```python
from build123d import *

# Parameters (mm, degrees)
SKETCH1_W                      = 60
SKETCH1_H                      = 375.5
BASE_FLANGE1_DEPTH             = 4
EDGE_FLANGE1_STRIP_W           = 18
EDGE_FLANGE1_STRIP_H           = 4
EDGE_FLANGE1_STRIP_CUT_DEPTH   = 375.5
EDGE_FLANGE1_DEPTH             = 375.5
EDGE_FLANGE2_STRIP_W           = 18
EDGE_FLANGE2_STRIP_H           = 4
EDGE_FLANGE2_STRIP_CUT_DEPTH   = 55
EDGE_FLANGE2_STRIP_2_W         = 18
EDGE_FLANGE2_STRIP_2_H         = 4
EDGE_FLANGE2_STRIP_CUT_2_DEPTH = 55
EDGE_FLANGE2_STRIP_3_W         = 18
EDGE_FLANGE2_STRIP_3_H         = 4
EDGE_FLANGE2_STRIP_CUT_3_DEPTH = 55
EDGE_FLANGE2_STRIP_4_W         = 18
EDGE_FLANGE2_STRIP_4_H         = 4
EDGE_FLANGE2_STRIP_CUT_4_DEPTH = 55
EDGE_FLANGE2_DEPTH             = 55
EDGE_FLANGE2_BEND_DEPTH        = 55
EDGE_FLANGE2_BEND_2_DEPTH      = 55
EDGE_FLANGE2_BEND_3_DEPTH      = 55
SKETCH18_R                     = 4.6
EXTRUDE1_DEPTH                 = 386.948506928
SKETCH19_R                     = 4.6
EXTRUDE2_DEPTH                 = 4
SKETCH20_R                     = 4.6
EXTRUDE3_DEPTH                 = 4


# Sheet-metal steps are written as plain solids
with BuildPart() as part:
    # Sketch1 → Base-Flange1 (new body)
    with BuildSketch(Plane(origin=(0, 0, 0), x_dir=(1, 0, 0), z_dir=(0, 1, 0))):
        Rectangle(SKETCH1_W, SKETCH1_H)
    extrude(amount=BASE_FLANGE1_DEPTH)

    # Edge-Flange1 strip (across the edge) → Edge-Flange1 strip cut (cut)
    with BuildSketch(Plane(origin=(-30, 4, -187.75), x_dir=(1, 0, 0), z_dir=(0, 0, 1))):
        with Locations((-4, -2)):
            Rectangle(EDGE_FLANGE1_STRIP_W, EDGE_FLANGE1_STRIP_H)
    extrude(amount=EDGE_FLANGE1_STRIP_CUT_DEPTH, mode=Mode.SUBTRACT)

    # Edge-Flange1 section (across the edge) → Edge-Flange1 (add)
    with BuildSketch(Plane(origin=(-30, 4, -187.75), x_dir=(1, 0, 0), z_dir=(0, 0, 1))):
        with BuildLine():
            Line((0, 1), (0, 56))
            Line((0, 56), (4, 56))
            Line((4, 56), (4, 1))
            ThreePointArc((4, 1), (4.292893219, 0.292893219), (5, 0))
            Line((5, 0), (5, -4))
            ThreePointArc((5, -4), (1.464466094, -2.535533906), (0, 1))
        make_face()
    extrude(amount=EDGE_FLANGE1_DEPTH)

    # Edge-Flange2 strip (across the edge) → Edge-Flange2 strip cut (cut)
    with BuildSketch(Plane(origin=(-30, 5, 187.75), x_dir=(0, 0, -1), z_dir=(0, 1, 0))):
        with Locations((-4, -2)):
            Rectangle(EDGE_FLANGE2_STRIP_W, EDGE_FLANGE2_STRIP_H)
    extrude(amount=EDGE_FLANGE2_STRIP_CUT_DEPTH, mode=Mode.SUBTRACT)

    # Edge-Flange2 strip 2 (across the edge) → Edge-Flange2 strip cut 2 (cut)
    with BuildSketch(Plane(origin=(30, 0, 187.75), x_dir=(0, 0, -1), z_dir=(-1, 0, 0))):
        with Locations((-4, -2)):
            Rectangle(EDGE_FLANGE2_STRIP_2_W, EDGE_FLANGE2_STRIP_2_H)
    extrude(amount=EDGE_FLANGE2_STRIP_CUT_2_DEPTH, mode=Mode.SUBTRACT)

    # Edge-Flange2 strip 3 (across the edge) → Edge-Flange2 strip cut 3 (cut)
    with BuildSketch(Plane(origin=(-30, 60, -187.75), x_dir=(0, 0, 1), z_dir=(0, -1, 0))):
        with Locations((-4, -2)):
            Rectangle(EDGE_FLANGE2_STRIP_3_W, EDGE_FLANGE2_STRIP_3_H)
    extrude(amount=EDGE_FLANGE2_STRIP_CUT_3_DEPTH, mode=Mode.SUBTRACT)

    # Edge-Flange2 strip 4 (across the edge) → Edge-Flange2 strip cut 4 (cut)
    with BuildSketch(Plane(origin=(-25, 0, -187.75), x_dir=(0, 0, 1), z_dir=(1, 0, 0))):
        with Locations((-4, -2)):
            Rectangle(EDGE_FLANGE2_STRIP_4_W, EDGE_FLANGE2_STRIP_4_H)
    extrude(amount=EDGE_FLANGE2_STRIP_CUT_4_DEPTH, mode=Mode.SUBTRACT)

    # Edge-Flange2 section (across the edge) → Edge-Flange2 (add)
    with BuildSketch(Plane(origin=(-30, 5, 187.75), x_dir=(0, 0, -1), z_dir=(0, 1, 0))):
        with BuildLine():
            Line((0, 1), (0, 36))
            Line((0, 36), (4, 36))
            Line((4, 36), (4, 1))
            ThreePointArc((4, 1), (4.292893219, 0.292893219), (5, 0))
            Line((5, 0), (5, -4))
            ThreePointArc((5, -4), (1.464466094, -2.535533906), (0, 1))
        make_face()
    extrude(amount=EDGE_FLANGE2_DEPTH)

    # Edge-Flange2 section 2 (across the edge) → Edge-Flange2 bend (add)
    with BuildSketch(Plane(origin=(30, 0, 187.75), x_dir=(0, 0, -1), z_dir=(-1, 0, 0))):
        with BuildLine():
            Line((0, 1), (0, 36))
            Line((0, 36), (4, 36))
            Line((4, 36), (4, 1))
            ThreePointArc((4, 1), (4.292893219, 0.292893219), (5, 0))
            Line((5, 0), (5, -4))
            ThreePointArc((5, -4), (1.464466094, -2.535533906), (0, 1))
        make_face()
    extrude(amount=EDGE_FLANGE2_BEND_DEPTH)

    # Edge-Flange2 section 3 (across the edge) → Edge-Flange2 bend 2 (add)
    with BuildSketch(Plane(origin=(-30, 60, -187.75), x_dir=(0, 0, 1), z_dir=(0, -1, 0))):
        with BuildLine():
            Line((0, 1), (0, 36))
            Line((0, 36), (4, 36))
            Line((4, 36), (4, 1))
            ThreePointArc((4, 1), (4.292893219, 0.292893219), (5, 0))
            Line((5, 0), (5, -4))
            ThreePointArc((5, -4), (1.464466094, -2.535533906), (0, 1))
        make_face()
    extrude(amount=EDGE_FLANGE2_BEND_2_DEPTH)

    # Edge-Flange2 section 4 (across the edge) → Edge-Flange2 bend 3 (add)
    with BuildSketch(Plane(origin=(-25, 0, -187.75), x_dir=(0, 0, 1), z_dir=(1, 0, 0))):
        with BuildLine():
            Line((0, 1), (0, 36))
            Line((0, 36), (4, 36))
            Line((4, 36), (4, 1))
            ThreePointArc((4, 1), (4.292893219, 0.292893219), (5, 0))
            Line((5, 0), (5, -4))
            ThreePointArc((5, -4), (1.464466094, -2.535533906), (0, 1))
        make_face()
    extrude(amount=EDGE_FLANGE2_BEND_3_DEPTH)

    # Sketch18 → Extrude1 (cut, through all)
    with BuildSketch(Plane.XY.offset(187.75)):
        with Locations((-46, 47.5)):
            Circle(SKETCH18_R)
        with Locations((-46, 17.5)):
            Circle(SKETCH18_R)
        with Locations((-12.5, -16)):
            Circle(SKETCH18_R)
        with Locations((17.5, -16)):
            Circle(SKETCH18_R)
    extrude(amount=-EXTRUDE1_DEPTH, mode=Mode.SUBTRACT)

    # Sketch19 → Extrude2 (cut)
    with BuildSketch(Plane(origin=(-26, 0, 0), x_dir=(0, 0, -1), z_dir=(1, 0, 0))):
        with Locations(Location((-107.75, 35, 0), (0, 0, 90))):
            Circle(SKETCH19_R)
        with Locations(Location((107.75, 35, 0), (0, 0, 90))):
            Circle(SKETCH19_R)
    extrude(amount=-EXTRUDE2_DEPTH, mode=Mode.SUBTRACT)

    # Sketch20 → Extrude3 (cut)
    with BuildSketch(Plane(origin=(0, 4, 0), x_dir=(1, 0, 0), z_dir=(0, 1, 0))):
        with Locations(Location((5, 107.75, 0), (0, 0, 270))):
            Circle(SKETCH20_R)
        with Locations(Location((5, -107.75, 0), (0, 0, 270))):
            Circle(SKETCH20_R)
    extrude(amount=-EXTRUDE3_DEPTH, mode=Mode.SUBTRACT)


solid = part.part
```
Model file for the job. Use its own axes, mm. A direction names the side the tool comes from. Coordinates: 2 decimals unless noted, no trailing zeros. Loops run counter-clockwise (first coordinate to the right, second up) from the corner with the lowest first, then second, coordinate; pieces in that order, holes last. Notation, with made-up numbers: (2, 74.5) - (23, 74.5) arc R13 cw to (23, 87.5) - close; hole circle Ø7 at (-12, -6.75). An arc over 180 degrees is marked (long way). Answer as a JSON object with one key per item and string values. Group by question number.
(1) Two-plate mould, pull along Y, no slides. Class faces 1 (the face through (-27.972, 37.123, -111.831)), 2 (the face through (-49, 33, -183.75)), 3 (the face through (-28, 60, 1)), 4 (the face through (-43.53, 21.38, -185.72)): released by +Y, released by -Y, zero draft, split by the parting line, or undercut.
(2) Flat gauge pins, fed straight in: pin 1 (12 mm diameter, centred on y = 35, z = 107.75, fed in from +X); pin 2 (1.5 mm diameter, centred on y = -11.5, z = -185.5, fed in from -X); pin 3 (3 mm diameter, centred on x = -18.5, z = 128.5, fed in from -Y). Where does each tip first touch, or does it go through?
(3) Cut at D-D (y = 17.5). Give the cut face in (x, z), then the cut area to 3 significant figures.
(4) Cut at C-C (x = -12.5). Give the cut face in (y, z), then the cut area to 3 significant figures.
(5) Tool access for faces 5 (the face through (-49, 32, 183.75)), 6 (the face through (-10.03, -12.12, 185.78)), 7 (the face through (2, 0, -3)): list every direction of +Z, -Z, +X, -X, +Y, -Y with a clear straight run to the whole face (end or side of a thin tool).
(6) Probe line 1 along Y through (x, z) = (-46, -185.95); line 2 along Z through (x, y) = (-9, -21); line 3 along X through (y, z) = (9, 117). List the from-to ranges inside material, lowest first.
(7) Cut at B-B (z = -107.75). Give the cut face in (x, y).
(8) Cut at A-A (y = -16). Give the cut face in (x, z), then the cut area to 3 significant figures.
Geometry says:
{
 "1": {"face 1": "undercut", "face 2": "zero draft", "face 3": "released by +Y", "face 4": "undercut"},
 "2": {"pin 1": "stops at x = -26", "pin 2": "stops at x = -25", "pin 3": "stops at y = 0"},
 "3": {"outline": "(-66, -187.75) - (-50.6, -187.75) - (-50.6, -183.75) - (-66, -183.75) - close; (-66, 183.75) - (-50.6, 183.75) - (-50.6, 187.75) - (-66, 187.75) - close; (-41.4, -187.75) - (-31, -187.75) arc R5 ccw to (-26, -182.75) - (-26, 182.75) arc R5 ccw to (-31, 187.75) - (-41.4, 187.75) - (-41.4, 183.75) - (-31, 183.75) arc R1 cw to (-30, 182.75) - (-30, -182.75) arc R1 cw to (-31, -183.75) - (-41.4, -183.75) - close", "area": "1,710 mm^2"},
 "4": {"outline": "(-36, -187.75) - (-20.6, -187.75) - (-20.6, -183.75) - (-36, -183.75) - close; (-36, 183.75) - (-20.6, 183.75) - (-20.6, 187.75) - (-36, 187.75) - close; (-11.4, -187.75) - (-1, -187.75) arc R5 ccw to (4, -182.75) - (4, 182.75) arc R5 ccw to (-1, 187.75) - (-11.4, 187.75) - (-11.4, 183.75) - (-1, 183.75) arc R1 cw to (0, 182.75) - (0, -182.75) arc R1 cw to (-1, -183.75) - (-11.4, -183.75) - close", "area": "1,710 mm^2"},
 "5": {"face 5": "-X, +Y, -Y", "face 6": "+Z, -Z", "face 7": "+X, -X, -Y"},
 "6": {"line 1": "y = 5 to 12.9, 22.1 to 42.9, 52.1 to 60", "line 2": "z = -187.75 to -183.75, 183.75 to 187.75", "line 3": "x = -30 to -26"},
 "7": {"outline": "(-30, 5) arc R5 ccw to (-25, 0) - (0.4, 0) - (0.4, 4) - (-25, 4) arc R1 cw to (-26, 5) - (-26, 30.4) - (-30, 30.4) - close; (-30, 39.6) - (-26, 39.6) - (-26, 60) - (-30, 60) - close; (9.6, 0) - (30, 0) - (30, 4) - (9.6, 4) - close"},
 "8": {"outline": "(-25, -187.75) - (-17.1, -187.75) - (-17.1, -183.75) - (-25, -183.75) - close; (-25, 183.75) - (-17.1, 183.75) - (-17.1, 187.75) - (-25, 187.75) - close; (-7.9, -187.75) - (12.9, -187.75) - (12.9, -183.75) - (-7.9, -183.75) - close; (-7.9, 183.75) - (12.9, 183.75) - (12.9, 187.75) - (-7.9, 187.75) - close; (22.1, -187.75) - (30, -187.75) - (30, -183.75) - (22.1, -183.75) - close; (22.1, 183.75) - (30, 183.75) - (30, 187.75) - (22.1, 187.75) - close", "area": "293 mm^2"}
}
